For this review, use the dimensioned drawing (mm, ordinates from the lowest corner) and the shaded views. A direction names the side the tool comes from. Coordinates: 2 decimals unless noted, no trailing zeros. Order: outer loops, then holes, each group sorted by start corner. A loop starts at its lowest first (then second) coordinate and runs counter-clockwise, first axis right, second up. Notation, with made-up numbers: M 59.5,67 L 73.5,67 A17 cw 73.5,92 Z; hole C 3.25,56.25 d4. An arc over 180 degrees is marked long. Answer in a Markdown table with one row per item.
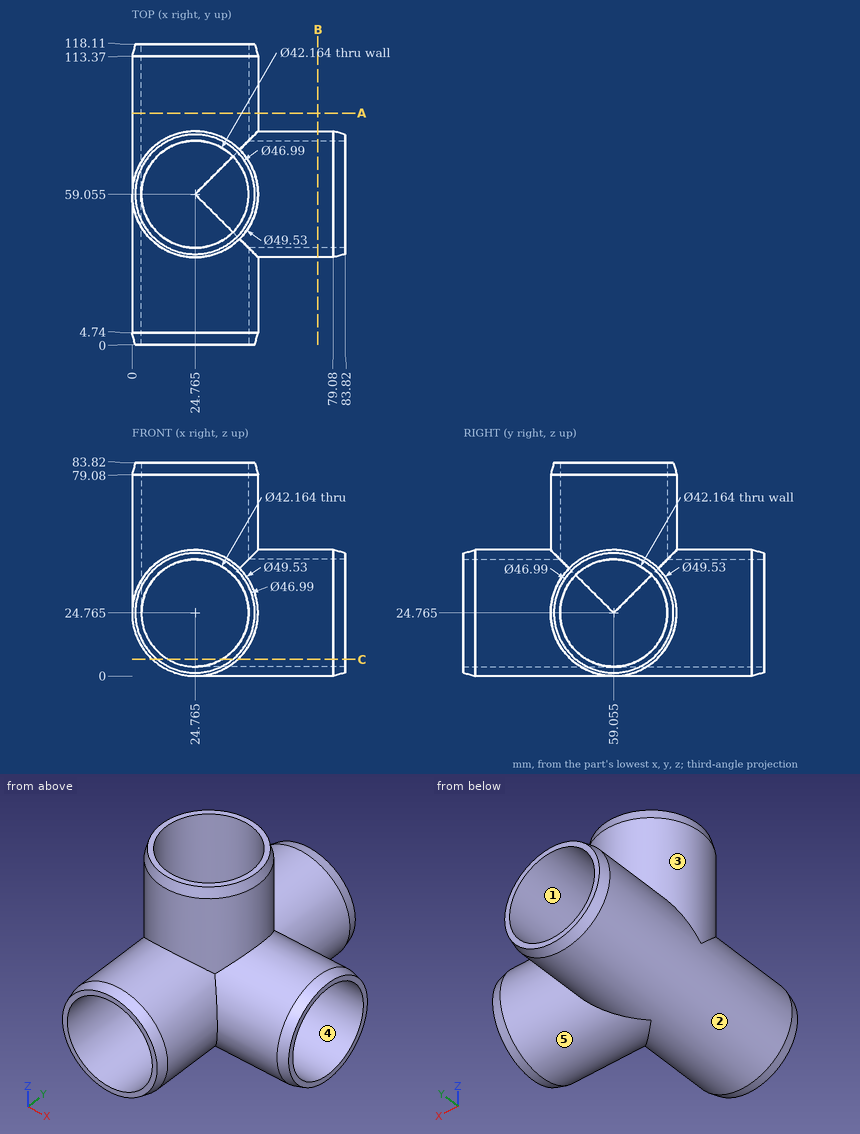
(1) For line 1 along Y through (x, z) = (71.5, 24.5) (1 decimal); line 2 along X through (y, z) = (100, 24); line 3 along Z through (x, y) = (32, 85.5), list the stretches that pass through material, from the lowest coordinate up. Write a range as from..to.
Return value:
| item | result |
|---|---|
| line 1 | y = 34.3..38, 80.1..83.8 |
| line 2 | x = 0.01..3.7, 45.83..49.52 |
| line 3 | z = 1.08..4.96, 44.57..48.45 |
(2) Draft analysis for pull direction Y (two halves, no side actions). For the marked faces 4 and 5, state which applies: pulls with the +Y half, pulls with the -Y half, needs draft (parallel to the pull), parting line crosses it, or undercut.
Return value:
| item | result |
|---|---|
| face 4 | undercut |
| face 5 | parting line crosses it |
(3) Insertion check: pin 1 Ø4 at (y, z) = (22.5, 26) entering from +X; pin 2 Ø5 at (y, z) = (43, 34) entering from -X; pin 3 Ø10 at (x, z) = (39.5, 72) entering from +Y. Each pin has a flat end and moves straight along its axis. Give the tip position at first contact, or say it passes through.
Return value:
| item | result |
|---|---|
| pin 1 | stops at x = 49.53 |
| pin 2 | stops at x = 0.93 |
| pin 3 | stops at y = 81.83 |
(4) Add section B-B, the plane x = 73. Give the boundary of the cut face in (y, z) (1 decimal).
Return value:
| item | result |
|---|---|
| outline | C 59.1,24.8 d49.5; hole C 59.1,24.8 d42.2 |
(5) For the marked faces 1, 2 and 3, list the 3-axis set-ups (+Z, -Z, +X, -X, +Y, -Y) from which the entire face can be reached by the end or side of a thin tool; tool diameter is ignored.
Return value:
| item | result |
|---|---|
| face 1 | +Y, -Y |
| face 2 | none |
| face 3 | +Z |
(6) Add section C-C, the plane z = 6.5. Give the number of separate pieces and of enclosed holes in the cut face, and give its area (3 significant figures).
Return value:
| item | result |
|---|---|
| separate pieces | 3 |
| enclosed holes | 0 |
| area | 1,830 mm2 |
(7) Add section A-A, the plane y = 91. Give the boundary of the cut face in (x, z) (1 decimal).
Return value:
| item | result |
|---|---|
| outline | C 24.8,24.8 d49.5; hole C 24.8,24.8 d42.2 |
